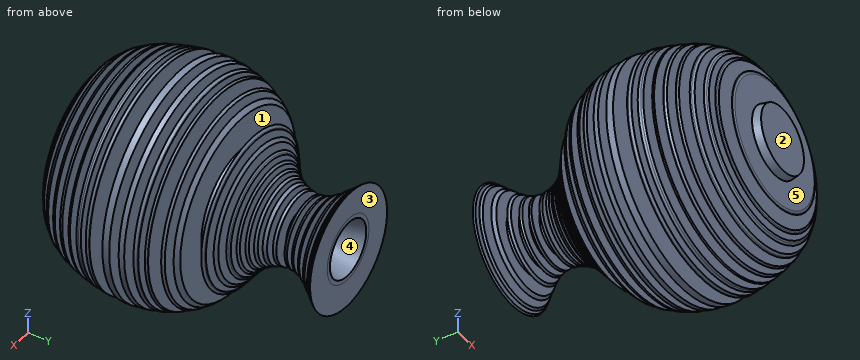
from build123d import *


with BuildPart() as f2:
    # F0 (on Top) → F2 (revolve)
    with BuildSketch(Plane.XY):
        Polygon((0, 9.378116), (0, 0), (24.604948, 0), (25.706446, 5.994941), (45.479894, 5.994941), (46.942912, 6.45127), (47.717456, 6.738137), (25.825249, 6.738137), (26.573369, 10.862892), (56.364384, 10.862892), (57.487395, 11.540667), (58.491852, 12.1359), (26.794957, 12.1359), (27.052034, 13.553292), (27.231239, 14.541335), (62.003512, 14.541335), (63.250378, 15.431428), (64.532876, 16.713921), (27.629765, 16.713921), (28.399006, 20.955124), (68.429738, 20.955124), (69.6574, 22.522839), (70.234209, 23.456283), (28.855346, 23.456283), (29.908466, 29.26265), (73.515236, 29.26265), (74.099392, 30.424284), (74.422076, 31.091657), (30.35906, 31.091657), (31.298541, 36.271477), (76.488361, 36.271477), (77.119462, 37.892114), (77.304818, 38.460255), (31.698201, 38.460255), (32.945067, 44.16668), (78.984402, 44.16668), (79.265952, 45.404524), (33.199325, 45.404524), (33.664483, 47.969166), (34.361847, 51.040873), (80.637857, 51.040873), (80.948345, 52.752745), (81.31466, 54.77242), (35.066795, 54.77242), (35.622962, 57.055045), (35.95968, 58.911538), (82.087442, 58.911538), (82.161032, 59.317274), (82.357049, 61.15666), (82.434862, 61.886843), (36.614653, 61.886843), (39.039336, 71.838244), (83.0843, 71.838244), (83.0843, 75.516842), (83.0843, 76.932549), (39.867867, 77.422731), (40.948308, 83.379733), (82.357049, 83.379733), (81.764966, 87.08635), (41.377679, 87.08635), (41.74902, 90.570949), (42.009386, 93.014168), (80.358267, 93.014168), (79.725832, 95.249459), (79.50262, 96.030705), (42.375591, 96.030705), (42.543257, 97.604053), (42.79562, 99.97218), (78.062922, 99.97218), (77.556342, 101.358041), (77.304818, 101.888739), (42.855736, 101.888739), (42.918192, 107.395157), (42.918192, 109.495983), (73.574463, 109.148265), (72.455429, 111.107185), (42.918192, 111.442211), (42.523887, 115.571633), (69.252551, 115.571633), (66.24417, 118.595034), (42.005457, 118.595034), (41.517783, 121.597573), (39.409656, 127.680138), (56.250583, 127.680138), (54.549944, 128.996819), (53.809993, 129.527852), (38.60588, 129.527852), (37.713028, 131.302819), (36.950387, 132.567689), (49.692087, 132.567689), (47.162347, 134.409189), (35.759922, 134.409189), (33.199325, 137.536392), (42.918192, 137.536392), (41.450825, 138.598174), (40.569924, 139.409781), (31.698201, 139.409781), (29.274845, 141.920537), (37.713028, 141.824827), (35.987534, 143.240124), (27.840512, 143.240124), (25.086587, 145.764545), (33.577848, 145.764545), (32.200888, 147.371009), (22.949941, 147.475938), (19.902222, 150.05295), (30.435741, 150.05295), (29.234551, 152.039543), (17.544426, 152.039543), (15.798809, 153.873503), (15.015064, 154.799744), (27.91124, 154.799744), (26.913745, 157.435983), (13.645455, 157.435983), (13.391357, 157.861903), (13.391357, 159.063086), (13.645455, 161.026582), (25.795961, 161.026582), (25.426364, 162.851468), (25.426364, 163.384512), (14.174428, 163.384512), (16.221292, 169.309467), (25.227502, 169.309467), (25.227502, 170.06506), (25.38457, 171.233371), (16.845074, 171.233371), (18.250721, 175.406411), (26.483802, 175.406411), (27.114909, 177.127615), (18.853141, 177.127615), (20.473117, 181.816533), (29.450566, 181.816533), (30.804308, 183.669016), (21.114364, 183.669016), (23.002477, 189.155236), (34.936786, 189.155236), (36.931772, 191.577718), (23.821849, 191.577718), (25.062887, 195.687234), (40.374566, 195.687234), (41.799556, 197.182268), (25.795961, 197.182268), (26.483802, 199.106008), (43.367047, 199.106008), (44.293292, 200.388506), (23.987159, 200.032249), (20.87367, 200.032249), (8.590471, 157.435983), (9.897195, 153.613403), (15.124086, 148.647845), (26.483802, 136.87174), (33.205751, 127.722636), (36.613557, 120.74475), (38.398597, 109.22312), (36.613557, 96.078731), (32.979747, 81.164822), (19.902222, 27.491957), (15.48874, 9.378116), align=None)
    revolve(axis=Axis((0, 101.371743, 0), (0, 1, 0)))


solid = f2.part
The listing builds one solid part. Answer for the finished solid, in the listing's coordinates (mm). Face numbers are marked on the shaded views. A direction names the side the tool comes from. Coordinates: 2 decimals unless noted, no trailing zeros. Loops run counter-clockwise (first coordinate to the right, second up) from the corner with the lowest first, then second, coordinate; pieces in that order, holes last.
1) Find section A-A on y = 166. Write down the section's boundary in (x, z), then the cut area to 3 significant figures.
2) Determine the mould class of the marked faces 4 and 5 for opening direction Z: pulls with the +Z half, pulls with the -Z half, needs draft (parallel to the pull), parting line crosses it, or undercut.
3) A tool of negligible diameter and unlimited length cuts with its end or side. For the marked faces 1, 2 and 3, from which of +Z, -Z, +X, -X, +Y, -Y can it reach the whole face along a straight path? Write none if from no direction.
4) Flat-ended cylindrical pins translate along their axes: pin 1 Ø24 at (x, z) = (11, -6.5) entering from +Y; pin 2 Ø12 at (x, z) = (-14.5, -14) entering from +Y; pin 3 Ø1 at (x, z) = (-27.5, 33) entering from -Y. Find the tip coordinate at first contact, or state that the pin passes through.
5) Find the intervals of material crossed by L1, parallel to X at y = 22, z = -13; L2, parallel to Z at x = 15, y = 91; L3, parallel to Z at x = -2, y = 61, in increasing order.
Values:
1. outline: circle Ø30.16 at (0, 0); hole circle Ø22.12 at (0, 0)
1. area: 330 mm2
2. face 4: undercut
2. face 5: needs draft
3. face 1: none
3. face 2: +Z, -Z, +X, -X, -Y
3. face 3: +Y
4. pin 1: stops at y = 200.05
4. pin 2: stops at y = 200.07
4. pin 3: stops at y = 5.99
5. L1: x = -68.02 to -13.25, 13.25 to 68.02
5. L2: z = -39.01 to -32.04, 32.04 to 39.01
5. L3: z = -82.32 to -28, 28 to 82.32
